Autodesk Inventor part; units mm, degrees
ref_plane "YZ Plane" through (0, 0, 0) normal (1, 0, 0) x (0, 1, 0)
ref_plane "XZ Plane" through (0, 0, 0) normal (0, 1, 0) x (-1, 0, 0)
ref_plane "XY Plane" through (0, 0, 0) normal (0, 0, 1) x (1, 0, 0)
sketch "Skizze1" plane through (0, 0, 0) normal (0, 0, 1) x (1, 0, 0)
  line L0 (0, 0) -> (12, 0)
  line L1 (12, 0) -> (12, 10)
  line L2 (12, 10) -> (0, 10)
  line L3 (0, 10) -> (0, 0)
  dimension "d0" = 12
  dimension "d1" = 10
extrude "Extrusion1" add sketch "Skizze1" along normal blind 14
sketch "Skizze2" plane through (0, 0, 14) normal (0, 0, 1) x (1, 0, 0)
  line L0 (1.05, 9.95) -> (10.95, 9.95)
  line L1 (10.95, 9.95) -> (10.95, 0.05)
  line L2 (10.95, 0.05) -> (1.05, 0.05)
  line L3 (1.05, 0.05) -> (1.05, 9.95)
  line L4 (12, 10) -> (0, 10)
  line L5 (0, 10) -> (0, 0)
  line L6 (0, 0) -> (12, 0)
  line L7 (0, 10) -> (12, 10)
  line L8 (12, 10) -> (12, 0)
  line L9 (12, 0) -> (0, 0)
  line L10 (0, 0) -> (0, 10)
  point P0 (6, 9.95)
  point P1 (6, 10)
  point P2 (1.05, 5)
  point P3 (0, 5)
  dimension "d4" = 9.9
  dimension "d5" = 9.9
extrude "Extrusion2" cut sketch "Skizze2" against normal blind 6.5
fillet "Rundung1" radius 2.1 4 edges at (1.05, 0.05, 10.75) (10.95, 0.05, 10.75) (10.95, 9.95, 10.75) (1.05, 9.95, 10.75)
fillet "Rundung2" radius 1 4 edges at (0, 0, 3.75) (0, 10, 3.75) (12, 0, 3.75) (12, 10, 3.75)
properties part number "Taster"
Model file for the job. Use its own axes, mm. A direction names the side the tool comes from. Coordinates: 2 decimals unless noted, no trailing zeros. Loops run counter-clockwise (first coordinate to the right, second up) from the corner with the lowest first, then second, coordinate; pieces in that order, holes last. Notation, with made-up numbers: (52, 25) -> (88, 25) arc R14 ccw to (88, 52) -> close; hole circle Ø9 at (73, 59.5). An arc over 180 degrees is marked (long way). Use one line per item in the form item = value. Start each with the question number.
(1) Flat gauge pins, fed straight in: pin 1 (4.5 mm diameter, centred on x = 5, z = 11, fed in from +Y); pin 2 (4.5 mm diameter, centred on y = 4.5, z = 10, fed in from +X). Where does each tip first touch, or does it go through?
(2) Probe probe 1 along Z at (x, y) = (0.5, 4.25); probe 2 along Y at (x, z) = (8.75, 12.25); probe 3 along X at (y, z) = (6.5, 8.25). List the from-to ranges inside material, lowest first. Write a range as from..to.
(3) Tool access for faces 1 (the flat face through (10.95, 5, 11)), 2 (the cylindrical face through (1.68, 0.65, 10.7)), 3 (the cylindrical face through (1.65, 9.32, 10.7)): list every direction of +Z, -Z, +X, -X, +Y, -Y with a clear straight run to the whole face (end or side of a thin tool).
(4) Cut at A-A on z = 8. Give the cut face in (x, y), and give its area (3 significant figures).
(5) Cut at B-B on y = 5.5. Give the cut face in (x, z), and give its area (3 significant figures).
Values:
q1.pin_1 = 9.95
q1.pin_2 = 10.95
q2.probe_1 = 0..7.5
q2.probe_2 = 0.05..9.95
q2.probe_3 = 1.05..10.95
q3.face_1 = +Z, +X, +Y, -Y
q3.face_2 = +Z, -X, -Y
q3.face_3 = +Z, -X, +Y
q4.outline = (1.05, 2.15) arc R2.1 ccw to (3.15, 0.05) -> (8.85, 0.05) arc R2.1 ccw to (10.95, 2.15) -> (10.95, 7.85) arc R2.1 ccw to (8.85, 9.95) -> (3.15, 9.95) arc R2.1 ccw to (1.05, 7.85) -> close
q4.area = 94.2 mm2
q5.outline = (0, 0) -> (12, 0) -> (12, 7.5) -> (10.95, 7.5) -> (10.95, 14) -> (1.05, 14) -> (1.05, 7.5) -> (0, 7.5) -> close
q5.area = 154 mm2
